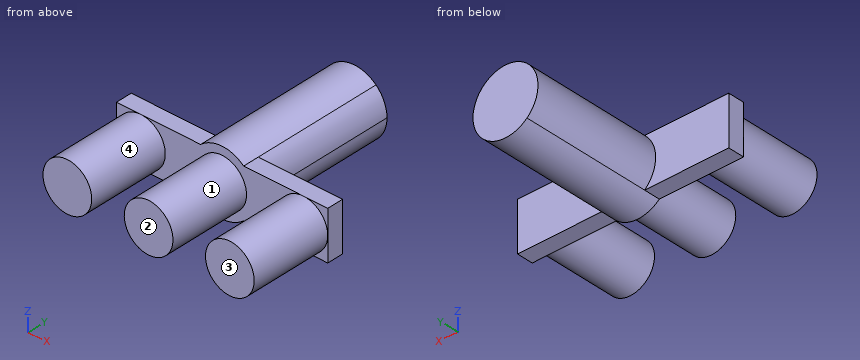
```python
from build123d import *

# Parameters (mm, degrees)
F1_DEPTH = 5
F2_DEPTH = 30
F3_DEPTH = 40


# Not quite as in the source:
# - after a boolean that leaves OpenCascade's solid faulty, fix() repairs it


with BuildPart() as f1:
    # F0 (on Front) → F1 (new body)
    with BuildSketch(Plane.XZ):
        with BuildLine():
            Line((-25, 7.5), (-32.5, 7.5))
            Line((-32.5, 7.5), (-32.5, 0))
            ThreePointArc((-32.5, 0), (-30.3033008589, 5.3033008589), (-25, 7.5))
        make_face()
        with BuildLine():
            Line((-6.6143782777, 7.5), (-25, 7.5))
            ThreePointArc((-25, 7.5), (-19.6966991411, 5.3033008589), (-17.5, 0))
            ThreePointArc((-17.5, 0), (-19.6966991411, -5.3033008589), (-25, -7.5))
            Line((-25, -7.5), (-6.6143782777, -7.5))
            ThreePointArc((-6.6143782777, -7.5), (-10, 0), (-6.6143782777, 7.5))
        make_face()
        with BuildLine():
            ThreePointArc((-17.5, 0), (-19.6966991411, 5.3033008589), (-25, 7.5))
            ThreePointArc((-25, 7.5), (-30.3033008589, 5.3033008589), (-32.5, 0))
            ThreePointArc((-32.5, 0), (-30.3033008589, -5.3033008589), (-25, -7.5))
            ThreePointArc((-25, -7.5), (-19.6966991411, -5.3033008589), (-17.5, 0))
        make_face()
        with BuildLine():
            ThreePointArc((-25, -7.5), (-30.3033008589, -5.3033008589), (-32.5, 0))
            Line((-32.5, 0), (-32.5, -7.5))
            Line((-32.5, -7.5), (-25, -7.5))
        make_face()
        with BuildLine():
            ThreePointArc((6.6143782777, 7.5), (0, 10), (-6.6143782777, 7.5))
            Line((-6.6143782777, 7.5), (0, 7.5))
            Line((0, 7.5), (6.6143782777, 7.5))
        make_face()
        with BuildLine():
            Line((0, 7.5), (-6.6143782777, 7.5))
            ThreePointArc((-6.6143782777, 7.5), (-10, 0), (-6.6143782777, -7.5))
            Line((-6.6143782777, -7.5), (-2.86e-08, -7.5))
            ThreePointArc((-2.86e-08, -7.5), (-7.5, 1.43e-08), (0, 7.5))
        make_face()
        with BuildLine():
            Line((6.6143782777, 7.5), (0, 7.5))
            ThreePointArc((0, 7.5), (5.3033008589, 5.3033008589), (7.5, 0))
            ThreePointArc((7.5, 0), (5.3033008488, -5.303300869), (-2.86e-08, -7.5))
            Line((-2.86e-08, -7.5), (6.6143782777, -7.5))
            ThreePointArc((6.6143782777, -7.5), (9.1143782777, -4.1143782777), (10, 0))
            ThreePointArc((10, 0), (9.1143782777, 4.1143782777), (6.6143782777, 7.5))
        make_face()
        with BuildLine():
            Line((25, 7.5), (6.6143782777, 7.5))
            ThreePointArc((6.6143782777, 7.5), (9.1143782777, 4.1143782777), (10, 0))
            ThreePointArc((10, 0), (9.1143782777, -4.1143782777), (6.6143782777, -7.5))
            Line((6.6143782777, -7.5), (25, -7.5))
            ThreePointArc((25, -7.5), (17.5, 0), (25, 7.5))
        make_face()
        with BuildLine():
            Line((-2.86e-08, -7.5), (-6.6143782777, -7.5))
            ThreePointArc((-6.6143782777, -7.5), (0, -10), (6.6143782777, -7.5))
            Line((6.6143782777, -7.5), (-2.86e-08, -7.5))
        make_face()
        with BuildLine():
            Line((32.5, 7.5), (25, 7.5))
            ThreePointArc((25, 7.5), (30.3033008589, 5.3033008589), (32.5, 0))
            Line((32.5, 0), (32.5, 7.5))
        make_face()
        with BuildLine():
            ThreePointArc((32.5, 0), (30.3033008589, 5.3033008589), (25, 7.5))
            ThreePointArc((25, 7.5), (17.5, 0), (25, -7.5))
            ThreePointArc((25, -7.5), (30.3033008589, -5.3033008589), (32.5, 0))
        make_face()
        with BuildLine():
            Line((32.5, -7.5), (32.5, 0))
            ThreePointArc((32.5, 0), (30.3033008589, -5.3033008589), (25, -7.5))
            Line((25, -7.5), (32.5, -7.5))
        make_face()
    extrude(amount=F1_DEPTH)

    # F0 (on Front) → F2 (join)
    with BuildSketch(Plane.XZ):
        with BuildLine():
            ThreePointArc((7.5, 0), (5.3033008589, 5.3033008589), (0, 7.5))
            ThreePointArc((0, 7.5), (-7.5, 1.43e-08), (-2.86e-08, -7.5))
            ThreePointArc((-2.86e-08, -7.5), (5.3033008488, -5.303300869), (7.5, 0))
        make_face()
        with BuildLine():
            ThreePointArc((32.5, 0), (30.3033008589, 5.3033008589), (25, 7.5))
            ThreePointArc((25, 7.5), (17.5, 0), (25, -7.5))
            ThreePointArc((25, -7.5), (30.3033008589, -5.3033008589), (32.5, 0))
        make_face()
        with BuildLine():
            ThreePointArc((-17.5, 0), (-19.6966991411, 5.3033008589), (-25, 7.5))
            ThreePointArc((-25, 7.5), (-30.3033008589, 5.3033008589), (-32.5, 0))
            ThreePointArc((-32.5, 0), (-30.3033008589, -5.3033008589), (-25, -7.5))
            ThreePointArc((-25, -7.5), (-19.6966991411, -5.3033008589), (-17.5, 0))
        make_face()
    extrude(amount=F2_DEPTH)

    # F0 (on Front) → F3 (join)
    with BuildSketch(Plane.XZ):
        with BuildLine():
            Line((0, 7.5), (-6.6143782777, 7.5))
            ThreePointArc((-6.6143782777, 7.5), (-10, 0), (-6.6143782777, -7.5))
            Line((-6.6143782777, -7.5), (-2.86e-08, -7.5))
            ThreePointArc((-2.86e-08, -7.5), (-7.5, 1.43e-08), (0, 7.5))
        make_face()
        with BuildLine():
            ThreePointArc((7.5, 0), (5.3033008589, 5.3033008589), (0, 7.5))
            ThreePointArc((0, 7.5), (-7.5, 1.43e-08), (-2.86e-08, -7.5))
            ThreePointArc((-2.86e-08, -7.5), (5.3033008488, -5.303300869), (7.5, 0))
        make_face()
        with BuildLine():
            Line((-2.86e-08, -7.5), (-6.6143782777, -7.5))
            ThreePointArc((-6.6143782777, -7.5), (0, -10), (6.6143782777, -7.5))
            Line((6.6143782777, -7.5), (-2.86e-08, -7.5))
        make_face()
        with BuildLine():
            Line((6.6143782777, 7.5), (0, 7.5))
            ThreePointArc((0, 7.5), (5.3033008589, 5.3033008589), (7.5, 0))
            ThreePointArc((7.5, 0), (5.3033008488, -5.303300869), (-2.86e-08, -7.5))
            Line((-2.86e-08, -7.5), (6.6143782777, -7.5))
            ThreePointArc((6.6143782777, -7.5), (9.1143782777, -4.1143782777), (10, 0))
            ThreePointArc((10, 0), (9.1143782777, 4.1143782777), (6.6143782777, 7.5))
        make_face()
        with BuildLine():
            ThreePointArc((6.6143782777, 7.5), (0, 10), (-6.6143782777, 7.5))
            Line((-6.6143782777, 7.5), (0, 7.5))
            Line((0, 7.5), (6.6143782777, 7.5))
        make_face()
    extrude(amount=-F3_DEPTH)

    add(f1.part.fix(), mode=Mode.REPLACE)


solid = f1.part
```
Source: CAD feature listing. Evaluate the final solid. Frame: model axes, mm. Face numbers are marked on the shaded views. A direction names the side the tool comes from. Coordinates: 2 decimals unless noted, no trailing zeros. Write each loop counter-clockwise with the first axis right and the second up, starting at its lowest first coordinate (ties: lowest second). Pieces come first, ordered by that corner, then holes. Notation, with made-up numbers: (68, 27.25) - (126, 27.25) arc R20 ccw to (126, 45.25) - close; hole circle Ø7 at (-10.5, 26.5). An arc over 180 degrees is marked (long way). Answer as a JSON object with one key per item and string values.
Q1. Section query B-B, the plane x = 0. Output: boundary loops of the cut face in (y, z).
Ans:
{"outline": "(-30, -7.5) - (-5, -7.5) - (-5, -10) - (40, -10) - (40, 10) - (-5, 10) - (-5, 7.5) - (-30, 7.5) - close"}
Q2. Section query A-A, the plane y = 30. Output: boundary loops of the cut face in (x, z), plus the area to 3 significant figures.
Ans:
{"outline": "circle Ø20 at (0, 0)", "area": "314 mm2"}
Q3. Set-up query: the marked faces 3 and 4. Return all of +Z, -Z, +X, -X, +Y, -Y with unobstructed straight access to the full face (end or side cutting, diameter ignored); none if empty.
Ans:
{"face 3": "+Z, -Z, +X, -X, -Y", "face 4": "-Y"}
Q4. Material intervals for line 1 (X direction, y = -9, z = -0.5); line 2 (X direction, y = -9, z = 6); line 3 (Y direction, x = -20.5, z = 3), sorted ascending. Write a range as [from, to].
Ans:
{"line 1": "x = [-32.48, -17.52], [-7.48, 7.48], [17.52, 32.48]", "line 2": "x = [-29.5, -20.5], [-4.5, 4.5], [20.5, 29.5]", "line 3": "y = [-30, 0]"}
Q5. Draft query along X for the marked faces 1 and 2. Return one class per face: released by +X, released by -X, zero draft, split by the parting line, or undercut.
Ans:
{"face 1": "undercut", "face 2": "zero draft"}
Q6. Section query D-D, the plane x = -12.5. Output: boundary loops of the cut face in (y, z).
Ans:
{"outline": "(-5, -7.5) - (0, -7.5) - (0, 7.5) - (-5, 7.5) - close"}
Q7. First-contact query: pin 1 Ø3 at (y, z) = (-11, 2.5) entering from -X; pin 2 Ø1.5 at (y, z) = (-7, 7.5) entering from +X; pin 3 Ø1 at (x, y) = (16, -5) entering from +Z. Flat tips, straight axial feed; report the tip coordinate or a pass-through.
Ans:
{"pin 1": "stops at x = -32.43", "pin 2": "stops at x = 28.27", "pin 3": "stops at z = 7.5"}
Q8. Section query C-C, the plane z = 3.25. Output: boundary loops of the cut face in (x, y).
Ans:
{"outline": "(-32.5, -5) - (-31.76, -5) - (-31.76, -30) - (-18.24, -30) - (-18.24, -5) - (-6.76, -5) - (-6.76, -30) - (6.76, -30) - (6.76, -5) - (18.24, -5) - (18.24, -30) - (31.76, -30) - (31.76, -5) - (32.5, -5) - (32.5, 0) - (9.46, 0) - (9.46, 40) - (-9.46, 40) - (-9.46, 0) - (-32.5, 0) - close"}
